from build123d import *

# Parameters (mm, degrees)
ESQUISSE1_W             = 120
ESQUISSE1_H             = 80
BOSS_EXTRU_1_DEPTH      = 5
ESQUISSE2_R             = 1.6
ENL_V_MAT_EXTRU_1_DEPTH = 145.308696897


with BuildPart() as part:
    # Esquisse1 → Boss.-Extru.1 (new body)
    with BuildSketch(Plane(origin=(0, 0, 0), x_dir=(1, 0, 0), z_dir=(0, 1, 0))):
        with Locations((60, 40)):
            Rectangle(ESQUISSE1_W, ESQUISSE1_H)
    extrude(amount=BOSS_EXTRU_1_DEPTH)

    # Esquisse2 → Enlèv. mat.-Extru.1 (cut, through all)
    with BuildSketch(Plane(origin=(0, 5, 0), x_dir=(1, 0, 0), z_dir=(0, 1, 0))):
        with Locations(Location((37.5, 67.5, 0), (0, 0, 270))):
            Circle(ESQUISSE2_R)
        with Locations(Location((82.5, 67.5, 0), (0, 0, 90))):
            Circle(ESQUISSE2_R)
        with Locations(Location((82.5, 12.5, 0), (0, 0, 270))):
            Circle(ESQUISSE2_R)
        with Locations(Location((37.5, 12.5, 0), (0, 0, 90))):
            Circle(ESQUISSE2_R)
        with Locations(Location((5, 75, 0), (0, 0, 270))):
            Circle(ESQUISSE2_R)
        with Locations(Location((115, 75, 0), (0, 0, 90))):
            Circle(ESQUISSE2_R)
        with Locations(Location((115, 5, 0), (0, 0, 270))):
            Circle(ESQUISSE2_R)
        with Locations(Location((5, 5, 0), (0, 0, 90))):
            Circle(ESQUISSE2_R)
        with BuildLine():
            Line((47.5, 70), (72.5, 70))
            ThreePointArc((72.5, 70), (75, 67.5), (72.5, 65))
            Line((72.5, 65), (47.5, 65))
            ThreePointArc((47.5, 65), (45, 67.5), (47.5, 70))
        make_face()
        with BuildLine():
            Line((47.5, 10), (72.5, 10))
            ThreePointArc((72.5, 10), (75, 12.5), (72.5, 15))
            Line((72.5, 15), (47.5, 15))
            ThreePointArc((47.5, 15), (45, 12.5), (47.5, 10))
        make_face()
    extrude(amount=-ENL_V_MAT_EXTRU_1_DEPTH, mode=Mode.SUBTRACT)


solid = part.part
Geometry: final body of the model. Coordinates: model frame, mm. A direction names the side the tool comes from. Give positions to 0.01 mm unless a question says otherwise; leave off trailing zeros. Write each loop counter-clockwise with the first axis right and the second up, starting at its lowest first coordinate (ties: lowest second). Pieces come first, ordered by that corner, then holes. Notation, with made-up numbers: M -29,-37.75 L -19,-37.75 A30 ccw -19,-9.75 Z; hole C 83.5,-33 d8. An arc over 180 degrees is marked long. Answer in a Markdown table with one row per item. Add a question column.
(1) Section C-C on y = 3.9. State how many separate pieces and enclosed holes the cut face has, and give its area (3 significant figures).
(2) Mould query, pull axis Z, two halves, no side actions, for faces 1 (the cylindrical face through (75, 2.5, -67.6)), 2 (the flat face through (59, 2, -80)), 3 (the flat face through (59, 2, 0)). Classes: +Z half, -Z half, draft (parallel to the pull), parting line (faces both ways), or undercut.
(3) Ray query, line 1 (Z direction, x = 60, y = 4.25); line 2 (X direction, y = 1.8, z = -12.5); line 3 (X direction, y = 2.75, z = -75). Return the intervals inside material, ascending.
(4) Section A-A on x = 57. Return loops of the section in (y, z), and give its area (3 significant figures).
(5) Reachability of faces 4 (the flat face through (59, 5, -41)), 5 (the flat face through (60, 3, -15)) from +Z, -Z, +X, -X, +Y, -Y: full face, straight path, thin tool, end or side. Return the list, or none.
(6) Section B-B on z = -5. Return loops of the section in (x, y), and give its area (3 significant figures).
Result set:
| question | item | result |
|---|---|---|
| 1 | separate pieces | 1 |
| 1 | enclosed holes | 10 |
| 1 | area | 9,250 mm^2 |
| 2 | face 1 | undercut |
| 2 | face 2 | -Z half |
| 2 | face 3 | +Z half |
| 3 | line 1 | z = -80 to -70, -65 to -15, -10 to 0 |
| 3 | line 2 | x = 0 to 35.9, 39.1 to 45, 75 to 80.9, 84.1 to 120 |
| 3 | line 3 | x = 0 to 3.4, 6.6 to 113.4, 116.6 to 120 |
| 4 | outline | M 0,-80 L 5,-80 L 5,-70 L 0,-70 Z; M 0,-65 L 5,-65 L 5,-15 L 0,-15 Z; M 0,-10 L 5,-10 L 5,0 L 0,0 Z |
| 4 | area | 350 mm^2 |
| 5 | face 4 | +Z, -Z, +X, -X, +Y |
| 5 | face 5 | +Y, -Y |
| 6 | outline | M 0,0 L 3.4,0 L 3.4,5 L 0,5 Z; M 6.6,0 L 113.4,0 L 113.4,5 L 6.6,5 Z; M 116.6,0 L 120,0 L 120,5 L 116.6,5 Z |
| 6 | area | 568 mm^2 |
